Work out the finished part from the listing and answer in its coordinate system (mm). Face numbers are marked on the shaded views. A direction names the side the tool comes from. Round coordinates to 2 decimals unless told otherwise and drop trailing zeros. Loops run counter-clockwise (first coordinate to the right, second up) from the corner with the lowest first, then second, coordinate; pieces in that order, holes last. Notation, with made-up numbers: M 46.5,57 L 68.5,57 A12 ccw 68.5,63 Z; hole C -16,-28 d2. An arc over 180 degrees is marked long. One line per item, written item: value.
Autodesk Inventor part; units mm, degrees
ref_plane "YZ Plane" through (0, 0, 0) normal (1, 0, 0) x (0, 1, 0)
ref_plane "XZ Plane" through (0, 0, 0) normal (0, 1, 0) x (-1, 0, 0)
ref_plane "XY Plane" through (0, 0, 0) normal (0, 0, 1) x (1, 0, 0)
sketch "Sketch7" plane through (0, 0, 0) normal (0, 0, 1) x (1, 0, 0)
  line L0 (0, 0) -> (100, 0)
  line L1 (100, 0) -> (100, -200)
  line L2 (100, -200) -> (0, -200)
  line L3 (0, -200) -> (0, 0)
  line L4 (100, 0) -> (80, 0)
  line L5 (80, 0) -> (80, -20)
  line L6 (80, -20) -> (100, -20)
  line L7 (100, -20) -> (100, 0)
  line L8 (100, -200) -> (80, -200)
  line L9 (80, -200) -> (80, -180)
  line L10 (80, -180) -> (100, -180)
  line L11 (100, -180) -> (100, -200)
  dimension "d23" = 100
  dimension "d24" = 200
  dimension "d25" = 20
  dimension "d26" = 20
extrude "Plate3" add sketch "Sketch7" along normal blind 3 contours L0 L5 L6 L1 L10 L9 L2 L3
sketch "Sketch8" plane through (0, 0, 3) normal (0, 0, 1) x (1, 0, 0)
  line L0 (6.2166, -35.2952) -> (70.6562, -35.2952) construction
  line L1 (70.6562, -35.2952) -> (70.6562, -48.8117) construction
  line L2 (70.6562, -48.8117) -> (6.2166, -48.8117) construction
  line L3 (6.2166, -48.8117) -> (6.2166, -35.2952) construction
  point P0 (0, 0)
mark "Mark2"
sketch "Sketch9" plane through (0, -200, 3) normal (0, 0, 1) x (1, 0, 0)
  circle A0 centre (25.6213, 34.9394) radius 13.2577
  point P0 (0, 200)
extrude "Cut1" cut sketch "Sketch9" against normal blind 3
sketch "Sketch10" plane through (0, 0, 0) normal (0, 0, -1) x (-1, 0, 0)
  line L0 (-87.8036, -108.5191) -> (-55.956, -108.5191) construction
  line L1 (-55.956, -108.5191) -> (-55.956, -118.5191) construction
  line L2 (-55.956, -118.5191) -> (-87.8036, -118.5191) construction
  line L3 (-87.8036, -118.5191) -> (-87.8036, -108.5191) construction
  point P0 (0, 0)
mark "Mark3"
sketch "Sketch11" plane through (97, -20, 0) normal (1, 0, 0) x (0, 1, 0)
  line L0 (-160, 0) -> (0, 0)
  line L1 (0, 0) -> (0, 25)
  line L2 (0, 25) -> (-160, 25)
  line L3 (-160, 25) -> (-160, 0)
edge flange "Flange2" height 25 angle 90 thickness 3 bend radius 5 thickness toward (1, 0, 0) relief round relief width 3 relief depth 1.5 edges at (100, -100, 3) wall of the first edge with corners at (97, -180, 0) (97, -20, 0) (97, -20, 25) (97, -180, 25)
bend "Bend2"
corner "Corner2"
equation "\"d28\" = Thickness"
equation "\"d27\" = Thickness"
equation "\"d30\" = BendReliefWidth"
equation "\"d31\" = BendReliefDepth"
equation "\"d32\" = MinimumRemnant"
equation "\"d33\" = TransitionRadius"
equation "\"d36\" = BendRadius"
equation "\"d37\" = CornerReliefSize"
equation "\"d38\" = GapSize"
equation "\"d39\" = JacobiRadiusSize"
equation "\"BendReliefWidth\" = Thickness"
equation "\"BendReliefDepth\" = 0.5 * Thickness"
equation "\"CornerReliefSize\" = 4 * Thickness"
equation "\"MinimumRemnant\" = 2 * Thickness"
equation "\"TransitionRadius\" = BendRadius"
equation "\"JacobiRadiusSize\" = BendRadius"
equation "\"GapSize\" = Thickness"
properties material "Stainless Steel"
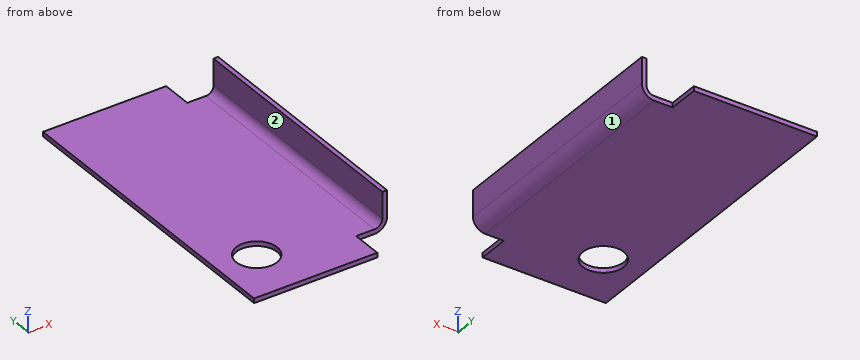
1) For the marked faces 1 and 2, determine the directions among +Z, -Z, +X, -X, +Y, -Y from which every point of the face is accessible in a straight line to the end or side of a thin tool.
Check values:
face 1: -Z, +X, +Y, -Y
face 2: +Z, -X, +Y, -Y
2) Find the intervals of material crossed by probe 1 along X at (y, z) = (-66, 13); probe 2 along Z at (x, y) = (73, -164.5); probe 3 along Y at (x, z) = (33, 1.75), in increasing order. Write a range as from..to.
Check values:
probe 1: 97..100
probe 2: 0..3
probe 3: -200..-176.08, -154.05..0
3) Find section A-A (x = 15). Give the vertices of the cut face in (y, z) (3 decimals).
Check values:
outline: M -200,0 L -172.995,0 L -172.995,3 L -200,3 Z; M -157.126,0 L 0,0 L 0,3 L -157.126,3 Z
4) Find section C-C (z = 13). Give the vertices of the cut face in (x, y).
Check values:
outline: M 97,-180 L 100,-180 L 100,-20 L 97,-20 Z
5) Each of these flat-tipped pins is pushed along its axis until it touches: pin 1 (13.5 mm diameter, centred on y = -124.5, z = 13.5, fed in from -X); pin 2 (0.9 mm diameter, centred on y = -11, z = 1.5, fed in from +X); pin 3 (4 mm diameter, centred on x = 59, y = -92.5, fed in from +Z). Where does it stop, or does it pass through?
Check values:
pin 1: x = 96.84
pin 2: x = 80
pin 3: z = 3
6) Find section D-D (x = 36.5). Give the vertices of the cut face in (y, z).
Check values:
outline: M -200,0 L -172.64,0 L -172.64,3 L -200,3 Z; M -157.48,0 L 0,0 L 0,3 L -157.48,3 Z
7) Find section B-B (y = -129). Give the vertices of the cut face in (x, z), then the cut area to 3 significant figures.
Check values:
outline: M 0,0 L 92,0 A8 ccw 100,8 L 100,25 L 97,25 L 97,8 A5 cw 92,3 L 0,3 Z
area: 358 mm2
